Check sheet for the drawn part. Datum: minimum x, y, z corner. Units: mm. A direction names the side the tool comes from. Round coordinates to 2 decimals unless told otherwise and drop trailing zeros. Write each loop counter-clockwise with the first axis right and the second up, starting at its lowest first coordinate (ties: lowest second). Pieces come first, ordered by that corner, then holes. Notation, with made-up numbers: (14, -11.75) -> (32, -11.75) arc R20 ccw to (32, 17.25) -> close; hole circle Ø3 at (-10.75, 8.5). An arc over 180 degrees is marked (long way). One line per item, written item: value.
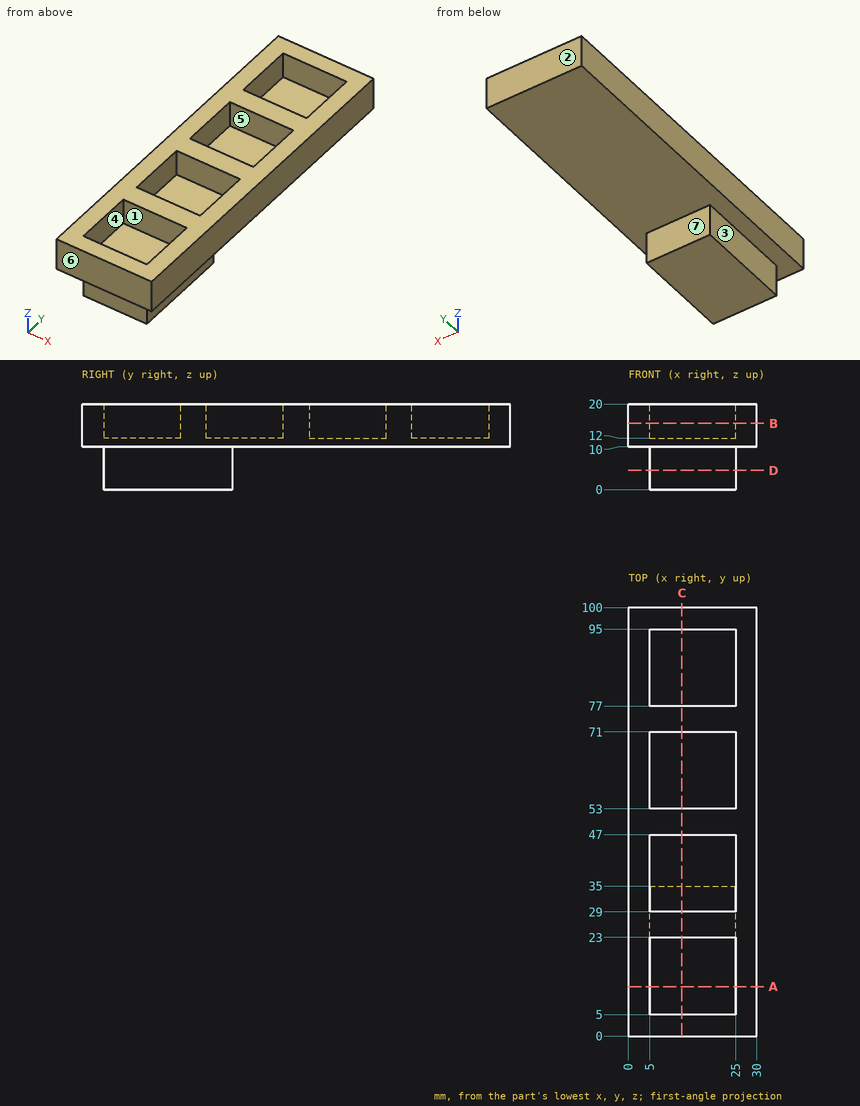
Item 1: Depth check by flat-ended pin: P1, Ø14.5, axis at x = 10.5, y = 90, coming from the +Z side; P2, Ø5, axis at x = 17, z = 6, coming from the +Y side; P3, Ø5, axis at x = 18.5, z = 6, coming from the -Y side; P4, Ø3, axis at x = 27, y = 39.5, coming from the -Z side. Enter the tip coordinate at first touch or a pass-through.
Answer:
P1: stops at z = 20
P2: stops at y = 35
P3: stops at y = 5
P4: stops at z = 10
Item 2: Sectioned sample at B-B on z = 15.5. Enter the section's corners in (x, y).
Answer:
outline: (0, 0) -> (30, 0) -> (30, 100) -> (0, 100) -> close; hole (5, 5) -> (25, 5) -> (25, 23) -> (5, 23) -> close; hole (5, 29) -> (25, 29) -> (25, 47) -> (5, 47) -> close; hole (5, 53) -> (25, 53) -> (25, 71) -> (5, 71) -> close; hole (5, 77) -> (25, 77) -> (25, 95) -> (5, 95) -> close
Item 3: Tool access check on the marked faces 5, 6 and 7. Record the directions out of +Z, -Z, +X, -X, +Y, -Y that give a thin tool (end or side, any length) a straight path to the whole face; none if there is none.
Answer:
face 5: +Z
face 6: +Z, -Z, +X, -X, -Y
face 7: -Z, +X, -X, +Y
Item 4: Sectioned sample at D-D on z = 4.5. Enter the section's corners in (x, y).
Answer:
outline: (5, 5) -> (25, 5) -> (25, 35) -> (5, 35) -> close
Item 5: Sectioned sample at A-A on y = 11.5. Enter the section's corners in (x, z).
Answer:
outline: (0, 10) -> (5, 10) -> (5, 0) -> (25, 0) -> (25, 10) -> (30, 10) -> (30, 20) -> (25, 20) -> (25, 12) -> (5, 12) -> (5, 20) -> (0, 20) -> close
Item 6: Thickness scan on line 1 (Y direction, x = 11, z = 17); line 2 (X direction, y = 62.5, z = 17.25); line 3 (Y direction, x = 6.5, z = 8). Record the ranges inside material, lowest first.
Answer:
line 1: y = 0 to 5, 23 to 29, 47 to 53, 71 to 77, 95 to 100
line 2: x = 0 to 5, 25 to 30
line 3: y = 5 to 35
Item 7: Sectioned sample at C-C on x = 12.5. Enter the section's corners in (y, z), and give its area (3 significant figures).
Answer:
outline: (0, 10) -> (5, 10) -> (5, 0) -> (35, 0) -> (35, 10) -> (100, 10) -> (100, 20) -> (95, 20) -> (95, 12) -> (77, 12) -> (77, 20) -> (71, 20) -> (71, 12) -> (53, 12) -> (53, 20) -> (47, 20) -> (47, 12) -> (29, 12) -> (29, 20) -> (23, 20) -> (23, 12) -> (5, 12) -> (5, 20) -> (0, 20) -> close
area: 724 mm^2
Item 8: Mould release check, pull along Y, two halves, no side actions. Record for the marked faces 1, 2, 3 and 4: pulls with the +Y half, pulls with the -Y half, needs draft (parallel to the pull), parting line crosses it, or undercut.
Answer:
face 1: undercut
face 2: pulls with the +Y half
face 3: needs draft
face 4: undercut
